Source: three-view drawing plus pictorial views. Frame: mm from the lowest corner of the part. A direction names the side the tool comes from. Give positions to 0.01 mm unless a question says otherwise; leave off trailing zeros. Order: outer loops, then holes, each group sorted by start corner. A loop starts at its lowest first (then second) coordinate and runs counter-clockwise, first axis right, second up. Notation, with made-up numbers: (1.25, 76.25) - (39.25, 76.25) arc R18 cw to (39.25, 90.25) - close; hole circle Ø5 at (14, 24). An arc over 180 degrees is marked (long way). Use CSV: the item, a comma, the result in double quotes.
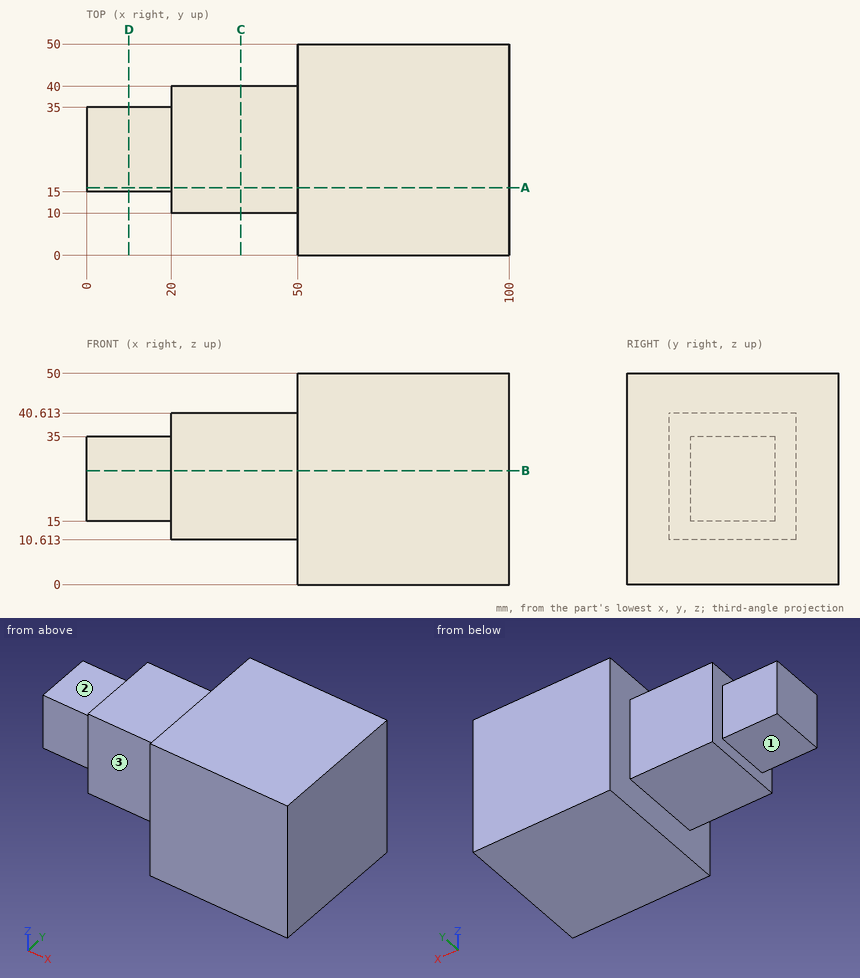
Item 1: Material intervals for line 1 (X direction, y = 42.5, z = 13); line 2 (Z direction, x = 25, y = 38.5); line 3 (Z direction, x = 13, y = 20.5), sorted ascending. Write a range as from..to.
Filled in:
line 1,"x = 50..100"
line 2,"z = 10.61..40.61"
line 3,"z = 15..35"
Item 2: Section C-C on x = 36.5. Return the cut outline in (y, z).
Filled in:
outline,"(10, 10.61) - (40, 10.61) - (40, 40.61) - (10, 40.61) - close"
Item 3: Set-up query: the marked faces 1, 2 and 3. Return all of +Z, -Z, +X, -X, +Y, -Y with unobstructed straight access to the full face (end or side cutting, diameter ignored); none if empty.
Filled in:
face 1,"-Z, -X, +Y, -Y"
face 2,"+Z, -X, +Y, -Y"
face 3,"+Z, -Z, -X, -Y"
Item 4: Section B-B on z = 27. Return the cut outline in (x, y).
Filled in:
outline,"(0, 15) - (20, 15) - (20, 10) - (50, 10) - (50, 0) - (100, 0) - (100, 50) - (50, 50) - (50, 40) - (20, 40) - (20, 35) - (0, 35) - close"
Item 5: Section A-A on y = 16. Return the cut outline in (x, z), then the cut area to 3 significant figures.
Filled in:
outline,"(0, 15) - (20, 15) - (20, 10.61) - (50, 10.61) - (50, 0) - (100, 0) - (100, 50) - (50, 50) - (50, 40.61) - (20, 40.61) - (20, 35) - (0, 35) - close"
area,"3,800 mm2"
Item 6: First-contact query: pin 1 (5 mm diameter, centred on x = 88.5, y = 9.5, fed in from -Z); pin 2 (1 mm diameter, centred on x = 49, y = 17.5, fed in from +Z); pin 3 (10 mm diameter, centred on x = 7.5, y = 28, fed in from -Z); pin 4 (6 mm diameter, centred on x = 16.5, y = 39, fed in from -Z). Flat tips, straight axial feed; report the tip coordinate or a pass-through.
Filled in:
pin 1,"stops at z = 0"
pin 2,"stops at z = 40.61"
pin 3,"stops at z = 15"
pin 4,"passes through"
Item 7: Section D-D on x = 10. Return the cut outline in (y, z), then the cut area to 3 significant figures.
Filled in:
outline,"(15, 15) - (35, 15) - (35, 35) - (15, 35) - close"
area,"400 mm2"
